Build history of the part. All positions in model axes, mm. A direction names the side the tool comes from. Give positions to 0.01 mm unless a question says otherwise; leave off trailing zeros. Write each question's results on one line, items separated by ' | '. Start each with the question number.
from build123d import *

# Parameters (mm, degrees)
SKETCH1_R           = 2.6035
BOSS_EXTRUDE1_DEPTH = 254


with BuildPart() as part:
    # Sketch1 → Boss-Extrude1 (new body)
    with BuildSketch(Plane(origin=(0, 0, -558.8), x_dir=(-1, 0, 0), z_dir=(0, 0, -1))):
        with BuildLine():
            Line((12.699999967, -9.5504), (12.699999967, -6.3246))
            ThreePointArc((12.699999967, -6.3246), (12.191999967, -5.8166), (12.699999967, -5.3086))
            Line((12.699999967, -5.3086), (12.699999967, 5.3086))
            ThreePointArc((12.699999967, 5.3086), (12.191999967, 5.8166), (12.699999967, 6.3246))
            Line((12.699999967, 6.3246), (12.699999967, 9.550399967))
            ThreePointArc((12.699999967, 9.550399967), (12.191999934, 10.058400016), (12.699999999, 10.566400033))
            ThreePointArc((12.699999999, 10.566400033), (12.082677404, 12.082677438), (10.566399999, 12.700000033))
            ThreePointArc((10.566399999, 12.700000033), (10.058400007, 12.192000016), (9.550399999, 12.700000016))
            Line((9.550399999, 12.700000016), (6.324599999, 12.700000016))
            ThreePointArc((6.324599999, 12.700000016), (5.816599999, 12.192000016), (5.308599999, 12.700000016))
            Line((5.308599999, 12.700000016), (4.302307888, 12.700000016))
            ThreePointArc((4.302307888, 12.700000016), (3.197407888, 11.595100016), (4.302307888, 10.490200016))
            Line((4.302307888, 10.490200016), (6.474794464, 10.490200016))
            ThreePointArc((6.474794464, 10.490200016), (7.413456072, 9.863006381), (7.193214956, 8.755779521))
            Line((7.193214956, 8.755779521), (3.875871421, 5.438435986))
            ThreePointArc((3.875871421, 5.438435986), (2.845827288, 4.7501825), (1.63080739, 4.508500016))
            Line((1.63080739, 4.508500016), (-1.630807376, 4.508500016))
            ThreePointArc((-1.630807376, 4.508500016), (-2.845827273, 4.7501825), (-3.875871406, 5.438435986))
            Line((-3.875871406, 5.438435986), (-7.193214947, 8.755779526))
            ThreePointArc((-7.193214947, 8.755779526), (-7.413456062, 9.863006383), (-6.474794457, 10.490200016))
            Line((-6.474794457, 10.490200016), (-4.302307919, 10.490200016))
            ThreePointArc((-4.302307919, 10.490200016), (-3.197407919, 11.595100016), (-4.302307919, 12.700000016))
            Line((-4.302307919, 12.700000016), (-5.308600001, 12.700000016))
            ThreePointArc((-5.308600001, 12.700000016), (-5.816600001, 12.192000016), (-6.324600001, 12.700000016))
            Line((-6.324600001, 12.700000016), (-9.550400001, 12.700000016))
            ThreePointArc((-9.550400001, 12.700000016), (-10.058400001, 12.192000016), (-10.566400001, 12.700000016))
            ThreePointArc((-10.566400001, 12.700000016), (-12.082677418, 12.082677417), (-12.700000017, 10.5664))
            ThreePointArc((-12.700000017, 10.5664), (-12.192, 10.058400008), (-12.7, 9.5504))
            Line((-12.7, 9.5504), (-12.7, 6.3246))
            ThreePointArc((-12.7, 6.3246), (-12.192, 5.8166), (-12.7, 5.3086))
            Line((-12.7, 5.3086), (-12.7, 4.302307889))
            ThreePointArc((-12.7, 4.302307889), (-11.5951, 3.197407889), (-10.4902, 4.302307889))
            Line((-10.4902, 4.302307889), (-10.4902, 6.474794456))
            ThreePointArc((-10.4902, 6.474794456), (-9.863006367, 7.413456061), (-8.75577951, 7.193214945))
            Line((-8.75577951, 7.193214945), (-5.43843597, 3.875871405))
            ThreePointArc((-5.43843597, 3.875871405), (-4.750182484, 2.845827272), (-4.5085, 1.630807374))
            Line((-4.5085, 1.630807374), (-4.5085, -1.630807374))
            ThreePointArc((-4.5085, -1.630807374), (-4.750182484, -2.845827272), (-5.43843597, -3.875871405))
            Line((-5.43843597, -3.875871405), (-8.75577951, -7.193214945))
            ThreePointArc((-8.75577951, -7.193214945), (-9.863006367, -7.413456061), (-10.4902, -6.474794456))
            Line((-10.4902, -6.474794456), (-10.4902, -4.302307918))
            ThreePointArc((-10.4902, -4.302307918), (-11.5951, -3.197407918), (-12.7, -4.302307918))
            Line((-12.7, -4.302307918), (-12.7, -5.3086))
            ThreePointArc((-12.7, -5.3086), (-12.192, -5.8166), (-12.7, -6.3246))
            Line((-12.7, -6.3246), (-12.7, -9.5504))
            ThreePointArc((-12.7, -9.5504), (-12.192, -10.058400008), (-12.700000017, -10.5664))
            ThreePointArc((-12.700000017, -10.5664), (-12.082677422, -12.082677406), (-10.566400017, -12.7))
            ThreePointArc((-10.566400017, -12.7), (-10.058400017, -12.192), (-9.550400017, -12.7))
            Line((-9.550400017, -12.7), (-6.324600017, -12.7))
            ThreePointArc((-6.324600017, -12.7), (-5.816600017, -12.192), (-5.308600017, -12.7))
            Line((-5.308600017, -12.7), (5.308599983, -12.7))
            ThreePointArc((5.308599983, -12.7), (5.816599983, -12.192), (6.324599983, -12.7))
            Line((6.324599983, -12.7), (9.550399983, -12.7))
            ThreePointArc((9.550399983, -12.7), (10.058399983, -12.192), (10.566399983, -12.7))
            ThreePointArc((10.566399983, -12.7), (12.082677389, -12.082677406), (12.699999983, -10.5664))
            ThreePointArc((12.699999983, -10.5664), (12.191999967, -10.058400008), (12.699999967, -9.5504))
        make_face()
        Circle(SKETCH1_R, mode=Mode.SUBTRACT)
        with BuildLine():
            Line((3.875871405, -5.43843597), (7.13192049, -8.694485055))
            ThreePointArc((7.13192049, -8.694485055), (7.35441848, -9.056211656), (7.4295, -9.4742))
            ThreePointArc((7.4295, -9.4742), (7.13192049, -10.19262049), (6.4135, -10.4902))
            Line((6.4135, -10.4902), (-6.4135, -10.4902))
            ThreePointArc((-6.4135, -10.4902), (-7.13192049, -10.19262049), (-7.4295, -9.4742))
            ThreePointArc((-7.4295, -9.4742), (-7.35441848, -9.056211656), (-7.13192049, -8.694485055))
            Line((-7.13192049, -8.694485055), (-3.875871405, -5.43843597))
            ThreePointArc((-3.875871405, -5.43843597), (-2.845827272, -4.750182484), (-1.630807374, -4.5085))
            Line((-1.630807374, -4.5085), (1.630807374, -4.5085))
            ThreePointArc((1.630807374, -4.5085), (2.845827272, -4.750182484), (3.875871405, -5.43843597))
        make_face(mode=Mode.SUBTRACT)
        with BuildLine():
            Line((10.490199999, 6.4135), (10.490199999, -6.413499984))
            ThreePointArc((10.490199999, -6.413499984), (10.192620488, -7.131920474), (9.474199999, -7.429499984))
            ThreePointArc((9.474199999, -7.429499984), (9.056211655, -7.354418464), (8.694485053, -7.131920474))
            Line((8.694485053, -7.131920474), (5.438435968, -3.875871389))
            ThreePointArc((5.438435968, -3.875871389), (4.750182483, -2.845827256), (4.508499999, -1.630807359))
            Line((4.508499999, -1.630807359), (4.508499999, 1.630807373))
            ThreePointArc((4.508499999, 1.630807373), (4.750182483, 2.845827271), (5.438435968, 3.875871403))
            Line((5.438435968, 3.875871403), (8.694485055, 7.13192049))
            ThreePointArc((8.694485055, 7.13192049), (9.056211656, 7.35441848), (9.4742, 7.4295))
            ThreePointArc((9.4742, 7.4295), (10.192620489, 7.131920489), (10.490199999, 6.4135))
        make_face(mode=Mode.SUBTRACT)
    extrude(amount=-BOSS_EXTRUDE1_DEPTH)


solid = part.part
Item 1: Cut at A-A, the plane z = -359.5. Count the separate pieces of the cut face and the enclosed holes in it, then the cut area to 3 significant figures.
Item 2: Probe line 1 along Y through (x, z) = (0, -492.5); line 2 along X through (y, z) = (-1, -530.5); line 3 along X through (y, z) = (7.25, -512.5). List the from-to ranges inside material, lowest first. Write a range as from..to.
Item 3: Which spindle directions (+Z, -Z, +X, -X, +Y, -Y) get a long thin tool onto all of the face, cutting with end or side? Do faces 4 (the flat face through (-3, 0, -304.8)), 5 (the flat face through (0, -10.49, -434)). Say none if no direction does.
Item 4: Two-plate mould, pull along X, no slides. Class faces 1 (the flat face through (-3, 0, -558.8)), 2 (the flat face through (-10.49, 0, -434)), 3 (the flat face through (-12.7, 0, -434)): +X half, -X half, draft (parallel to the pull), parting line (faces both ways), or undercut.
Item 5: Flat gauge pins, fed straight in: pin 1 Ø1 at (x, y) = (4, -8.5) entering from +Z; pin 2 Ø4 at (x, z) = (0, -456.5) entering from +Y; pin 3 Ø3 at (x, z) = (-2.5, -486) entering from +Y. Where does each tip first touch, or does it go through?
Values found:
1) separate pieces: 1 | enclosed holes: 3 | area: 311 mm2
2) line 1: y = -12.7..-10.49, -4.51..-2.6, 2.6..4.51 | line 2: x = -12.7..-10.49, -4.51..-2.4, 2.4..4.51 | line 3: x = -12.7..-10.05, -8.85..-5.69, 5.69..8.82, 10.13..12.7
3) face 4: +Z, +X, -X, +Y, -Y | face 5: +Z, -Z
4) face 1: draft | face 2: undercut | face 3: -X half
5) pin 1: passes through | pin 2: stops at y = 4.53 | pin 3: stops at y = 12.66
